```python
from build123d import *

# Parameters (mm, degrees)
F1_DEPTH = 20
F2_R     = 9.99999
F3_R     = 5
F4_DEPTH = 30


# Not quite as in the source:
# - a fillet or chamfer is up to 0.001 mm smaller than in the source, because OpenCascade refuses the exact size


with BuildPart() as f1:
    # F0 (on Right) → F1 (new body)
    with BuildSketch(Plane.YZ):
        with BuildLine():
            Line((-80, 0), (0, 0))
            Line((0, 0), (0, 40))
            Line((0, 40), (-19.1886116992, 40))
            ThreePointArc((-19.1886116992, 40), (-19.9895229142, 39.9354372882), (-20.7697505292, 39.7434164903))
            Line((-20.7697505292, 39.7434164903), (-76.5811388301, 21.13962039))
            ThreePointArc((-76.5811388301, 21.13962039), (-79.0562109259, 19.319755323), (-80, 16.3962038997))
            Line((-80, 16.3962038997), (-80, 0))
        make_face()
    extrude(amount=F1_DEPTH)

    # F2 (radius 10 in the source; OpenCascade refuses exactly that, so slightly less here)
    f2_edges = [f1.edges().sort_by_distance(p)[0] for p in [
        (20, -40, 0),
        (0, -40, 0),
    ]]
    fillet(f2_edges, radius=F2_R)

    # F3 (on face) → F4 (join)
    with BuildSketch(Plane(origin=(0, 0, 0), x_dir=(-1, 0, 0), z_dir=(0, 1, 0))):
        with Locations((-10, 10)):
            Circle(F3_R)
    extrude(amount=F4_DEPTH)


solid = f1.part
```
Here's how the part is built. I have some questions about the finished solid (model axes, mm). A direction names the side the tool comes from. Coordinates: 2 decimals unless noted, no trailing zeros. Write each loop counter-clockwise with the first axis right and the second up, starting at its lowest first coordinate (ties: lowest second). Pieces come first, ordered by that corner, then holes. Notation, with made-up numbers: (-37, 37.5) - (-12, 37.5) arc R30 cw to (-12, 60.5) - close; hole circle Ø6 at (-23, -9.75). An arc over 180 degrees is marked (long way). One line per item, written item: value.
1) I'm going to push flat-ended pins straight in: P1, Ø10, axis at x = 10.5, z = 26.5, coming from the +Y side; P2, Ø6, axis at x = 8.5, y = -57.5, coming from the +Z side; P3, Ø2, axis at x = 7, y = -35, coming from the +Z side. Where does each tip first touch, or does it pass through?
Model answer:
P1: stops at y = 0
P2: stops at z = 28.5
P3: stops at z = 35.33
2) On a 3-axis mill with a long thin cutter (end or side, diameter ignored), from which of +Z, -Z, +X, -X, +Y, -Y can I reach the whole of each face in a straight line? I mean faces 1 (the cylindrical face through (5.23, 14.79, 11.5)), 2 (the cylindrical face through (9.86, -79.03, 19.355)). Say none if no direction works.
Model answer:
face 1: +Y
face 2: +Z, +X, -X, -Y
3) Suppose I cut it at A-A on x = 2. Write out the boundary of the cut face in (y, z).
Model answer:
outline: (-80, 4) - (0, 4) - (0, 40) - (-19.19, 40) arc R5 ccw to (-20.77, 39.74) - (-76.58, 21.14) arc R5 ccw to (-80, 16.4) - close
4) I need wall thicknesses on line 1 along Y through (x, z) = (2.75, 9); line 2 along Z through (x, y) = (9.5, -8.5); line 3 along Z through (x, y) = (5, -61). Which ranges of each line are inside material? Lowest first, please.
Model answer:
line 1: y = -80 to 0
line 2: z = 0.01 to 40
line 3: z = 1.34 to 26.33
5) Suppose I cut it at B-B on z = 13.5. Write out the boundary of the cut face in (x, y).
Model answer:
outline: (0, -80) - (20, -80) - (20, 0) - (13.57, 0) - (13.57, 30) - (6.43, 30) - (6.43, 0) - (0, 0) - close
